Geometry: final body of the model. Coordinates: model frame, mm. Face numbers are marked on the shaded views. A direction names the side the tool comes from. Coordinates: 2 decimals unless noted, no trailing zeros. Write each loop counter-clockwise with the first axis right and the second up, starting at its lowest first coordinate (ties: lowest second). Pieces come first, ordered by that corner, then holes. Notation, with made-up numbers: M 69.25,40.25 L 110.25,40.25 A36 cw 110.25,76.25 Z; hole C 16,19 d11. An arc over 180 degrees is marked long. Write item = value, one per line. Start each with the question number.
Item 1: Section C-C on x = -1.5. Output: boundary loops of the cut face in (y, z), plus the area to 3 significant figures.
Item 2: Section D-D on x = 14. Output: boundary loops of the cut face in (y, z).
Item 3: First-contact query: pin 1 Ø2 at (x, z) = (28, -2) entering from +Y. Flat tip, straight axial feed; report the tip coordinate or a pass-through.
Item 4: Section B-B on x = -30. Output: boundary loops of the cut face in (y, z).
Item 5: Reachability of the marked faces 1 and 2 from +Z, -Z, +X, -X, +Y, -Y: full face, straight path, thin tool, end or side. Return the list, or none.
Item 6: Section A-A on z = 14. Output: boundary loops of the cut face in (x, y), plus the area to 4 significant figures.
Item 7: Pull-direction query (Z, two-part tool) for the marked faces 3, 4 and 5; classes: +Z half, -Z half, draft (parallel to the pull), parting line (faces both ways), or undercut.
Item 8: Ray query, L1, parallel to X at y = 0.7, z = 0; L2, parallel to X at y = 17, z = -24.5; L3, parallel to Z at x = 18, y = 23. Return the intervals inside material, ascending. Write a range as [from, to].
from build123d import *

# Parameters (mm, degrees)
CROQUIS_CONTORNO_W            = 110
CROQUIS_CONTORNO_H            = 65
CUERPO_DEPTH                  = 40
CROQUIS_VACIADO_W             = 105
CROQUIS_VACIADO_H             = 60
VACIADO_DEPTH                 = 37.5
CROQUIS_APOYOS_PCB_W          = 6
CROQUIS_APOYOS_PCB_H          = 6
APOYOS_PCB_DEPTH              = 6
CROQUIS_SALIDAS_W             = 13
CROQUIS_SALIDAS_H             = 8
CROQUIS_SALIDAS_W_2           = 11
CROQUIS_SALIDAS_H_2           = 7
SALIDAS_USB_Y_PANEL_DEPTH     = 76.374067158
VENTILAS_LATERALES_DEPTH      = 76.374067158
VENTILAS_LATERALES_DEPTH_BACK = 76.374067158
AGUJEROS_M3_DEPTH             = 76.374067158
AGUJEROS_M3_DEPTH_BACK        = 76.374067158
CROQUIS_TORNILLOS_R           = 1.7


with BuildPart() as part:
    # Croquis_contorno → Cuerpo (new body)
    with BuildSketch(Plane(origin=(0, 0, 0), x_dir=(1, 0, 0), z_dir=(0, 1, 0))):
        Rectangle(CROQUIS_CONTORNO_W, CROQUIS_CONTORNO_H)
    extrude(amount=CUERPO_DEPTH)

    # Croquis_vaciado → Vaciado (cut)
    with BuildSketch(Plane(origin=(0, 40, 0), x_dir=(1, 0, 0), z_dir=(0, 1, 0))):
        Rectangle(CROQUIS_VACIADO_W, CROQUIS_VACIADO_H)
    extrude(amount=-VACIADO_DEPTH, mode=Mode.SUBTRACT)

    # Croquis_apoyos_pcb → Apoyos_PCB (add)
    with BuildSketch(Plane(origin=(0, 2.5, 0), x_dir=(1, 0, 0), z_dir=(0, 1, 0))):
        with Locations((-41, 22)):
            Rectangle(CROQUIS_APOYOS_PCB_W, CROQUIS_APOYOS_PCB_H)
        with Locations((-41, -22)):
            Rectangle(CROQUIS_APOYOS_PCB_W, CROQUIS_APOYOS_PCB_H)
        with Locations((41, 22)):
            Rectangle(CROQUIS_APOYOS_PCB_W, CROQUIS_APOYOS_PCB_H)
        with Locations((41, -22)):
            Rectangle(CROQUIS_APOYOS_PCB_W, CROQUIS_APOYOS_PCB_H)
    extrude(amount=APOYOS_PCB_DEPTH)

    # Croquis_salidas → Salidas_USB_y_panel (cut, through all)
    with BuildSketch(Plane.XY):
        with Locations((9.3, 21.7)):
            Rectangle(CROQUIS_SALIDAS_W, CROQUIS_SALIDAS_H)
        with Locations((-13.46, 15.1)):
            Rectangle(CROQUIS_SALIDAS_W_2, CROQUIS_SALIDAS_H_2)
    extrude(amount=-SALIDAS_USB_Y_PANEL_DEPTH, mode=Mode.SUBTRACT)

    # Croquis_ventilas → Ventilas_laterales (cut, two sides: drawn at the far end of the back side and taken through both)
    with BuildSketch(Plane(origin=(0, 0, 0), x_dir=(0, 0, -1), z_dir=(1, 0, 0)).offset(-VENTILAS_LATERALES_DEPTH_BACK)):
        with BuildLine():
            Line((-15.2, 16.2), (-15.2, 33.8))
            ThreePointArc((-15.2, 33.8), (-14, 35), (-12.8, 33.8))
            Line((-12.8, 33.8), (-12.8, 16.2))
            ThreePointArc((-12.8, 16.2), (-14, 15), (-15.2, 16.2))
        make_face()
        with BuildLine():
            Line((-8.2, 16.2), (-8.2, 33.8))
            ThreePointArc((-8.2, 33.8), (-7, 35), (-5.8, 33.8))
            Line((-5.8, 33.8), (-5.8, 16.2))
            ThreePointArc((-5.8, 16.2), (-7, 15), (-8.2, 16.2))
        make_face()
        with BuildLine():
            Line((-1.2, 16.2), (-1.2, 33.8))
            ThreePointArc((-1.2, 33.8), (0, 35), (1.2, 33.8))
            Line((1.2, 33.8), (1.2, 16.2))
            ThreePointArc((1.2, 16.2), (0, 15), (-1.2, 16.2))
        make_face()
        with BuildLine():
            Line((5.8, 16.2), (5.8, 33.8))
            ThreePointArc((5.8, 33.8), (7, 35), (8.2, 33.8))
            Line((8.2, 33.8), (8.2, 16.2))
            ThreePointArc((8.2, 16.2), (7, 15), (5.8, 16.2))
        make_face()
        with BuildLine():
            Line((12.8, 16.2), (12.8, 33.8))
            ThreePointArc((12.8, 33.8), (14, 35), (15.2, 33.8))
            Line((15.2, 33.8), (15.2, 16.2))
            ThreePointArc((15.2, 16.2), (14, 15), (12.8, 16.2))
        make_face()
    extrude(amount=VENTILAS_LATERALES_DEPTH + VENTILAS_LATERALES_DEPTH_BACK, mode=Mode.SUBTRACT)

    # Croquis_tornillos → Agujeros_M3 (cut, two sides: drawn at the far end of the back side and taken through both)
    with BuildSketch(Plane(origin=(0, 0, 0), x_dir=(1, 0, 0), z_dir=(0, 1, 0)).offset(-AGUJEROS_M3_DEPTH_BACK)):
        with Locations(Location((-30, 0, 0), (0, 0, 90))):
            Circle(CROQUIS_TORNILLOS_R)
        with Locations(Location((30, 0, 0), (0, 0, 90))):
            Circle(CROQUIS_TORNILLOS_R)
    extrude(amount=AGUJEROS_M3_DEPTH + AGUJEROS_M3_DEPTH_BACK, mode=Mode.SUBTRACT)


solid = part.part
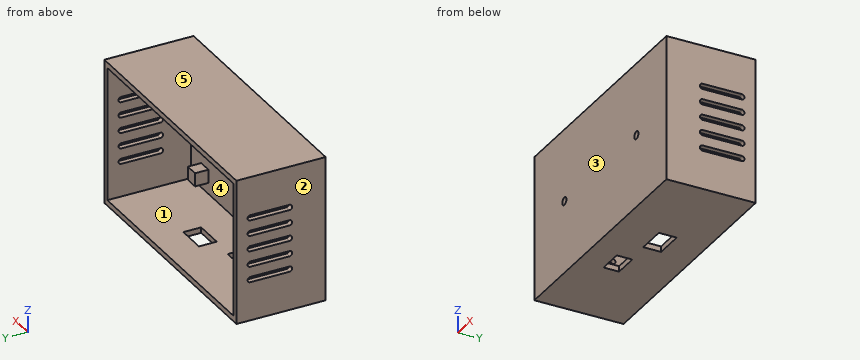
Responses:
q1.outline = M 0,-32.5 L 40,-32.5 L 40,-30 L 2.5,-30 L 2.5,30 L 40,30 L 40,32.5 L 0,32.5 Z
q1.area = 350 mm²
q2.outline = M 0,-32.5 L 17.7,-32.5 L 17.7,-30 L 2.5,-30 L 2.5,30 L 40,30 L 40,32.5 L 0,32.5 Z; M 25.7,-32.5 L 40,-32.5 L 40,-30 L 25.7,-30 Z
q3.pin_1 = 2.5
q4.outline = M 0,-32.5 L 40,-32.5 L 40,-30 L 2.5,-30 L 2.5,-1.7 L 0,-1.7 Z; M 0,1.7 L 2.5,1.7 L 2.5,30 L 40,30 L 40,32.5 L 0,32.5 Z
q5.face_1 = +Y
q5.face_2 = +Z, -Z, -X, +Y, -Y
q6.outline = M -55,0 L 55,0 L 55,15 L 52.5,15 L 52.5,2.5 L -52.5,2.5 L -52.5,15 L -55,15 Z; M -55,35 L -52.5,35 L -52.5,40 L -55,40 Z; M 52.5,35 L 55,35 L 55,40 L 52.5,40 Z
q6.area = 362.5 mm²
q7.face_3 = draft
q7.face_4 = undercut
q7.face_5 = +Z half
q8.L1 = [-55, -31.7], [-28.3, 28.3], [31.7, 55]
q8.L2 = [-55, -52.5], [52.5, 55]
q8.L3 = [-32.5, -30], [30, 32.5]
